Work out the finished part from the listing and answer in its coordinate system (mm). Face numbers are marked on the shaded views. A direction names the side the tool comes from. Coordinates: 2 decimals unless noted, no trailing zeros. Order: outer loops, then holes, each group sorted by start corner. A loop starts at its lowest first (then second) coordinate and runs counter-clockwise, first axis right, second up. Notation, with made-up numbers: (-18, 59) -> (22, 59) arc R26 ccw to (22, 85) -> close; hole circle Ø2 at (82, 31.25). An arc over 180 degrees is marked (long way). Use one line per item in the form item = value.
from build123d import *

# Parameters (mm, degrees)
SKETCH1_R           = 4.4
SKETCH1_R_2         = 2.5
BOSS_EXTRUDE1_DEPTH = 2.1
CUT_EXTRUDE1_DEPTH  = 1.27
SKETCH3_R           = 2.5
BOSS_EXTRUDE2_DEPTH = 36


with BuildPart() as part:
    # Sketch1 → Boss-Extrude1 (new body)
    # profile 1 of 2: a face of its own
    with BuildSketch(Plane(origin=(0, 0, 0), x_dir=(1, 0, 0), z_dir=(0, 1, 0))):
        with Locations(Location((0, 0, 0), (0, 0, 270))):
            Circle(SKETCH1_R)
        Circle(SKETCH1_R_2, mode=Mode.SUBTRACT)
    # profile 2 of 2: a face of its own
    with BuildSketch(Plane(origin=(0, 0, 0), x_dir=(1, 0, 0), z_dir=(0, 1, 0))):
        Circle(SKETCH1_R_2)
    extrude(amount=BOSS_EXTRUDE1_DEPTH)

    # Sketch2 → Cut-Extrude1 (cut)
    with BuildSketch(Plane.XZ):
        Polygon((2.886751346, 0), (1.443375673, 2.5), (-1.443375673, 2.5), (-2.886751346, 0), (-1.443375673, -2.5), (1.443375673, -2.5), align=None)
    extrude(amount=-CUT_EXTRUDE1_DEPTH, mode=Mode.SUBTRACT)

    # Sketch3 → Boss-Extrude2 (add)
    with BuildSketch(Plane(origin=(0, 2.1, 0), x_dir=(1, 0, 0), z_dir=(0, 1, 0))):
        with Locations(Location((0, 0, 0), (0, 0, 270))):
            Circle(SKETCH3_R)
    extrude(amount=BOSS_EXTRUDE2_DEPTH)


solid = part.part
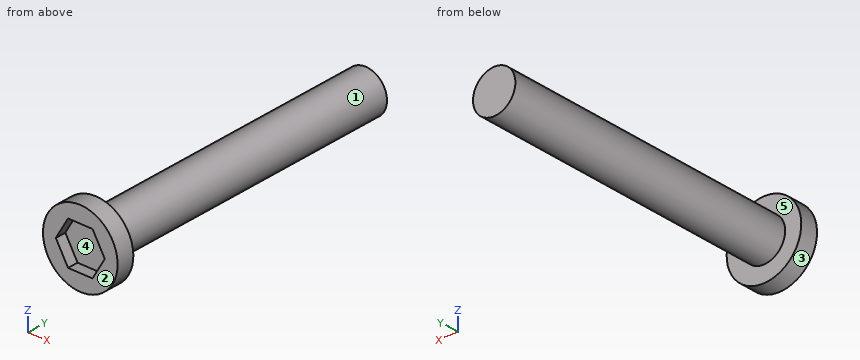
(1) Section A-A on x = 0 is taken. Write down the section's boundary in (y, z), plus the area to 3 significant figures.
Data:
outline = (0, -4.4) -> (2.1, -4.4) -> (2.1, -2.5) -> (38.1, -2.5) -> (38.1, 2.5) -> (2.1, 2.5) -> (2.1, 4.4) -> (0, 4.4) -> (0, 2.5) -> (1.27, 2.5) -> (1.27, -2.5) -> (0, -2.5) -> close
area = 192 mm²
(2) Which of the six approach directions +Z, -Z, +X, -X, +Y, -Y give full straight-line access (tool end or side, diameter ignored) to the marked faces 1 and 2?
Data:
face_1 = +Y
face_2 = +Z, -Z, +X, -X, -Y
(3) Section D-D on x = 4 is taken. Write down the section's boundary in (y, z).
Data:
outline = (0, -1.83) -> (2.1, -1.83) -> (2.1, 1.83) -> (0, 1.83) -> close
(4) The mould has two halves that part along X. Classify the marked faces 3, 4 and 5: released by +X, released by -X, zero draft, split by the parting line, or undercut.
Data:
face_3 = split by the parting line
face_4 = undercut
face_5 = zero draft
(5) Section C-C on y = 30.5 is taken. Write down the section's boundary in (x, z), plus the area to 3 significant figures.
Data:
outline = circle Ø5 at (0, 0)
area = 19.6 mm²
(6) Each of these flat-tipped pins is pushed along its axis until it touches: P1, Ø1.5, axis at y = 17, z = -1, coming from the +X side; P2, Ø2.5, axis at x = 0.5, z = 0.5, coming from the -Y side; P3, Ø2, axis at x = -3, z = -2, coming from the +Y side. Where does it stop, or does it pass through?
Data:
P1 = 2.49
P2 = 1.27
P3 = 2.1
(7) Straight lines are drawn through the part: line 1 along Y through (x, z) = (-0.75, -0.5); line 2 along Y through (x, z) = (3, -2.5); line 3 along X through (y, z) = (18.5, 1). For each, find the intervals that lie inside material, in ascending order.
Data:
line_1 = 1.27 to 38.1
line_2 = 0 to 2.1
line_3 = -2.29 to 2.29
(8) Section B-B on z = -0.5 is taken. Write down the section's boundary in (x, y), plus the area to 3 significant figures.
Data:
outline = (-4.37, 0) -> (-2.6, 0) -> (-2.6, 1.27) -> (2.6, 1.27) -> (2.6, 0) -> (4.37, 0) -> (4.37, 2.1) -> (2.45, 2.1) -> (2.45, 38.1) -> (-2.45, 38.1) -> (-2.45, 2.1) -> (-4.37, 2.1) -> close
area = 188 mm²
